The model under review builds one solid part; all positions refer to its coordinate system, in mm. A direction names the side the tool comes from. Round coordinates to 2 decimals unless told otherwise and drop trailing zeros. Loops run counter-clockwise (first coordinate to the right, second up) from the corner with the lowest first, then second, coordinate; pieces in that order, holes last. Notation, with made-up numbers: M 62.25,-27 L 90.25,-27 A15 cw 90.25,-12 Z; hole C 22,26 d4. An arc over 180 degrees is marked long. Answer as a JSON object with one key per item and string values. Group by question number.
Item 1: Insertion check: P1, Ø4, axis at x = 30.5, y = -8.5, coming from the -Z side; P2, Ø14.5, axis at y = -12.7, z = 31.75, coming from the +X side; P3, Ø12.5, axis at x = 67.5, y = -10.5, coming from the +Z side; P4, Ø10, axis at y = -18.5, z = 5, coming from the +X side. Each pin has a flat end and moves straight along its axis. Give the tip position at first contact, or say it passes through.
Item 2: Consider section C-C (y = -18). Give the boundary of the cut face in (x, z).
Item 3: Tool access review of faces 1 (the face through (62.12, -18.9, 6.44)), 2 (the face through (67, -7, 12.7)), 3 (the face through (25.4, -13, 25)): name each direction out of +Z, -Z, +X, -X, +Y, -Y from which nothing blocks a thin tool from reaching the whole face with its end or side.
Item 4: The part is to be moulded in two halves that separate along Y. For faces 4 (the face through (38, -25.4, 14)), 5 (the face through (19, -10, 12.7)), 6 (the face through (7.66, -16.56, 6.44)), say which applies: +Y half, -Y half, draft (parallel to the pull), parting line (faces both ways), or undercut.
Item 5: Consider section A-A (x = 12.7). Give the boundary of the cut face in (y, z), and give its area (3 significant figures).
Item 6: To check wall thickness, follow line 1 (Y direction, x = 63.5, z = 9.5); line 2 (X direction, y = -7, z = 5); line 3 (X direction, y = -9.5, z = 9.5). State the ranges of each line that lie inside material, in increasing order.
Item 7: Consider section D-D (z = 31.75). Give the boundary of the cut face in (x, y).
Item 8: Consider section B-B (z = 11.5). Give the boundary of the cut face in (x, y) (3 decimals), and give its area (3 significant figures).
```python
from build123d import *

# Parameters (mm, degrees)
F1_DEPTH  = 25.4
F2_R      = 6.35
F3_DEPTH  = 25.4
F5_DEPTH  = 25.4
F6_R      = 6.35
F7_DEPTH  = 25.4
F8_R      = 6.35
F9_DEPTH  = 25.4
F11_DEPTH = 25.4
F13_DEPTH = 25.4


with BuildPart() as f1:
    # F0 (on Front) → F1 (new body)
    with BuildSketch(Plane.XZ):
        Polygon((0, 12.7), (0, 0), (76.2, 0), (76.2, 12.7), (50.8, 12.7), (50.8, 44.45), (25.4, 44.45), (25.4, 12.7), align=None)
    extrude(amount=F1_DEPTH)

    # F2 (on face) → F3 (cut)
    with BuildSketch(Plane.YZ.offset(50.8)):
        with Locations((-12.7, 31.75)):
            Circle(F2_R)
    extrude(amount=-F3_DEPTH, mode=Mode.SUBTRACT)

    # F4 (on face) → F5 (cut)
    with BuildSketch(Plane.YZ.offset(50.8)):
        with BuildLine():
            ThreePointArc((-25.4, 34.29), (-20.8319677815, 41.5974597269), (-12.7, 44.45))
            Line((-12.7, 44.45), (-25.4, 44.45))
            Line((-25.4, 44.45), (-25.4, 34.29))
        make_face()
        with BuildLine():
            ThreePointArc((-12.7, 44.45), (-4.5680322185, 41.5974597269), (0, 34.29))
            Line((0, 34.29), (0, 44.45))
            Line((0, 44.45), (-12.7, 44.45))
        make_face()
    extrude(amount=-F5_DEPTH, mode=Mode.SUBTRACT)

    # F6 (on face) → F7 (cut)
    with BuildSketch(Plane.XY.offset(12.7)):
        with Locations((63.5, -12.7)):
            Circle(F6_R)
    extrude(amount=-F7_DEPTH, mode=Mode.SUBTRACT)

    # F8 (on face) → F9 (cut)
    with BuildSketch(Plane.XY.offset(12.7)):
        with Locations((12.7, -12.7)):
            Circle(F8_R)
    extrude(amount=-F9_DEPTH, mode=Mode.SUBTRACT)

    # F10 (on face) → F11 (cut)
    with BuildSketch(Plane.XY.offset(12.7)):
        with BuildLine():
            ThreePointArc((66.5324394711, 0), (73.5081244057, -4.719528106), (76.2, -12.6999999989))
            Line((76.2, -12.6999999989), (76.2, 0))
            Line((76.2, 0), (66.5324394711, 0))
        make_face()
        with BuildLine():
            ThreePointArc((76.2, -12.6999999989), (73.5081244064, -20.6804718932), (66.5324394711, -25.4))
            Line((66.5324394711, -25.4), (76.2, -25.4))
            Line((76.2, -25.4), (76.2, -12.6999999989))
        make_face()
    extrude(amount=-F11_DEPTH, mode=Mode.SUBTRACT)

    # F12 (on face) → F13 (cut)
    with BuildSketch(Plane.XY.offset(12.7)):
        with BuildLine():
            ThreePointArc((9.5950094983, -25.4), (0.2534522323, -12.8279951022), (9.240250381, 0))
            Line((9.240250381, 0), (0, 0))
            Line((0, 0), (0, -25.4))
            Line((0, -25.4), (9.5950094983, -25.4))
        make_face()
    extrude(amount=-F13_DEPTH, mode=Mode.SUBTRACT)


solid = f1.part
```
Geometry results:
{
 "1": {"P1": "stops at z = 0", "P2": "stops at x = 50.8", "P3": "stops at z = 12.7", "P4": "stops at x = 76.18"},
 "2": {"outline": "M 1.37,0 L 9.2,0 L 9.2,12.7 L 1.37,12.7 Z; M 16.2,0 L 60,0 L 60,12.7 L 50.8,12.7 L 50.8,28.25 L 25.4,28.25 L 25.4,12.7 L 16.2,12.7 Z; M 25.4,35.25 L 50.8,35.25 L 50.8,43.32 L 25.4,43.32 Z; M 67,0 L 75.09,0 L 75.09,12.7 L 67,12.7 Z"},
 "3": {"face 1": "+Z, -Z", "face 2": "+Z, +X, +Y, -Y", "face 3": "+Z, -X, +Y, -Y"},
 "4": {"face 4": "-Y half", "face 5": "draft", "face 6": "undercut"},
 "5": {"outline": "M -25.4,0 L -19.05,0 L -19.05,12.7 L -25.4,12.7 Z; M -6.35,0 L 0,0 L 0,12.7 L -6.35,12.7 Z", "area": "161 mm^2"},
 "6": {"line 1": "y = -25.4 to -19.05, -6.35 to 0", "line 2": "x = 1.5 to 9.9, 15.5 to 60.7, 66.3 to 74.9", "line 3": "x = 0.63 to 7.22, 18.18 to 58.02, 68.98 to 75.81"},
 "7": {"outline": "M 25.4,-25.4 L 50.8,-25.4 L 50.8,-19.05 L 25.4,-19.05 Z; M 25.4,-6.35 L 50.8,-6.35 L 50.8,0 L 25.4,0 Z"},
 "8": {"outline": "M 9.24,0 A13.383 ccw 9.595,-25.4 L 66.532,-25.4 A13.176 ccw 66.532,0 Z; hole C 12.7,-12.7 d12.7; hole C 63.5,-12.7 d12.7", "area": "1,550 mm^2"}
}
